The model under review builds one solid part; all positions refer to its coordinate system, in mm. A direction names the side the tool comes from. Give positions to 0.01 mm unless a question says otherwise; leave off trailing zeros. Order: outer loops, then holes, each group sorted by start corner. A loop starts at its lowest first (then second) coordinate and runs counter-clockwise, first axis right, second up. Notation, with made-up numbers: (3.25, 66.25) -> (14.25, 66.25) arc R28 ccw to (14.25, 93.25) -> close; hole circle Ø4 at (66, -18). An arc over 180 degrees is marked (long way). Answer as a JSON object with one key per item and string values. Group by question number.
from build123d import *

# Parameters (mm, degrees)
SKETCH_3_R           = 9.5
CUT_EXTRUDE_1_DEPTH  = 321.526909947
SKETCH_4_R           = 9.5
CUT_EXTRUDE_2_DEPTH  = 321.526909947
SKETCH_5_R           = 9.5
CUT_EXTRUDE_3_DEPTH  = 321.526909947
SKETCH_6_R           = 9.5
CUT_EXTRUDE_4_DEPTH  = 321.526909947
SKETCH_7_R           = 9.5
CUT_EXTRUDE_5_DEPTH  = 321.526909947
SKETCH_8_R           = 9.5
CUT_EXTRUDE_6_DEPTH  = 321.526909947
SKETCH_9_R           = 9.5
CUT_EXTRUDE_7_DEPTH  = 321.526909947
SKETCH_10_R          = 9.5
CUT_EXTRUDE_8_DEPTH  = 321.526909947
SKETCH_11_R          = 9.5
CUT_EXTRUDE_9_DEPTH  = 321.526909947
SKETCH_12_R          = 9.5
CUT_EXTRUDE_10_DEPTH = 321.526909947
SKETCH_13_R          = 9.5
CUT_EXTRUDE_11_DEPTH = 321.526909947
SKETCH_14_R          = 9.5
CUT_EXTRUDE_12_DEPTH = 321.526909947


with BuildPart() as part:
    # Эскиз1 → Повернуть1 (revolve)
    with BuildSketch(Plane.XY, mode=Mode.PRIVATE) as revolve_1_sk:
        Polygon((0, 0), (265, 0), (265, 127.5), (239, 127.5), (239, 100), (239, 95), (220, 95), (220, 94), (200, 94), (144, 65.5), (70, 65.5), (25, 41), (1.5, 41), (3, 45), (0, 45), align=None)
    revolve(revolve_1_sk.sketch.rotate(Axis((0, 0, 0), (1, 0, 0)), 90), axis=Axis((0, 0, 0), (1, 0, 0)))

    # Эскиз2 → Вырез-Повернуть1 (revolve, cut)
    with BuildSketch(Plane.XY, mode=Mode.PRIVATE) as cut_revolve_1_sk:
        with BuildLine():
            Line((0, 0), (200, 0))
            Line((200, 0), (200, 55))
            Line((200, 55), (192.669873, 55))
            ThreePointArc((192.669873, 55), (191.273625348, 54.108499061), (191.669873, 52.5))
            Line((191.669873, 52.5), (188.5, 52.5))
            ThreePointArc((188.5, 52.5), (187.75, 52.602347572), (187, 52.5))
            Line((187, 52.5), (177, 52.5))
            Line((177, 52.5), (95, 52.5))
            Line((95, 52.5), (90, 52.5))
            ThreePointArc((90, 52.5), (79.13262933, 46.740617582), (70, 38.502577))
            Line((70, 38.502577), (42, 31))
            Line((42, 31), (0, 31))
            Line((0, 31), (0, 0))
        make_face()
    revolve(cut_revolve_1_sk.sketch.rotate(Axis((0, 0, 0), (1, 0, 0)), 90), axis=Axis((0, 0, 0), (1, 0, 0)), mode=Mode.SUBTRACT)

    # Эскиз3 → Вырез-Вытянуть1 (cut, through all)
    with BuildSketch(Plane(origin=(0, 0, 0), x_dir=(0, 0, -1), z_dir=(1, 0, 0))):
        with Locations((0, 113)):
            Circle(SKETCH_3_R)
    extrude(amount=CUT_EXTRUDE_1_DEPTH, mode=Mode.SUBTRACT)

    # Эскиз4 → Вырез-Вытянуть2 (cut, through all)
    with BuildSketch(Plane(origin=(0, 0, 0), x_dir=(0, 0, -1), z_dir=(1, 0, 0))):
        with Locations((-56.5, 97.860870628)):
            Circle(SKETCH_4_R)
    extrude(amount=CUT_EXTRUDE_2_DEPTH, mode=Mode.SUBTRACT)

    # Эскиз5 → Вырез-Вытянуть3 (cut, through all)
    with BuildSketch(Plane(origin=(0, 0, 0), x_dir=(0, 0, -1), z_dir=(1, 0, 0))):
        with Locations((-97.860870628, 56.5)):
            Circle(SKETCH_5_R)
    extrude(amount=CUT_EXTRUDE_3_DEPTH, mode=Mode.SUBTRACT)

    # Эскиз6 → Вырез-Вытянуть4 (cut, through all)
    with BuildSketch(Plane(origin=(0, 0, 0), x_dir=(0, 0, -1), z_dir=(1, 0, 0))):
        with Locations((-113, 0)):
            Circle(SKETCH_6_R)
    extrude(amount=CUT_EXTRUDE_4_DEPTH, mode=Mode.SUBTRACT)

    # Эскиз7 → Вырез-Вытянуть5 (cut, through all)
    with BuildSketch(Plane(origin=(0, 0, 0), x_dir=(0, 0, -1), z_dir=(1, 0, 0))):
        with Locations((-97.860870628, -56.5)):
            Circle(SKETCH_7_R)
    extrude(amount=CUT_EXTRUDE_5_DEPTH, mode=Mode.SUBTRACT)

    # Эскиз8 → Вырез-Вытянуть6 (cut, through all)
    with BuildSketch(Plane(origin=(0, 0, 0), x_dir=(0, 0, -1), z_dir=(1, 0, 0))):
        with Locations((-56.5, -97.860870628)):
            Circle(SKETCH_8_R)
    extrude(amount=CUT_EXTRUDE_6_DEPTH, mode=Mode.SUBTRACT)

    # Эскиз9 → Вырез-Вытянуть7 (cut, through all)
    with BuildSketch(Plane(origin=(0, 0, 0), x_dir=(0, 0, -1), z_dir=(1, 0, 0))):
        with Locations((0, -113)):
            Circle(SKETCH_9_R)
    extrude(amount=CUT_EXTRUDE_7_DEPTH, mode=Mode.SUBTRACT)

    # Эскиз10 → Вырез-Вытянуть8 (cut, through all)
    with BuildSketch(Plane(origin=(0, 0, 0), x_dir=(0, 0, -1), z_dir=(1, 0, 0))):
        with Locations((56.5, -97.860870628)):
            Circle(SKETCH_10_R)
    extrude(amount=CUT_EXTRUDE_8_DEPTH, mode=Mode.SUBTRACT)

    # Эскиз11 → Вырез-Вытянуть9 (cut, through all)
    with BuildSketch(Plane(origin=(0, 0, 0), x_dir=(0, 0, -1), z_dir=(1, 0, 0))):
        with Locations((97.860870628, -56.5)):
            Circle(SKETCH_11_R)
    extrude(amount=CUT_EXTRUDE_9_DEPTH, mode=Mode.SUBTRACT)

    # Эскиз12 → Вырез-Вытянуть10 (cut, through all)
    with BuildSketch(Plane(origin=(0, 0, 0), x_dir=(0, 0, -1), z_dir=(1, 0, 0))):
        with Locations((113, 0)):
            Circle(SKETCH_12_R)
    extrude(amount=CUT_EXTRUDE_10_DEPTH, mode=Mode.SUBTRACT)

    # Эскиз13 → Вырез-Вытянуть11 (cut, through all)
    with BuildSketch(Plane(origin=(0, 0, 0), x_dir=(0, 0, -1), z_dir=(1, 0, 0))):
        with Locations((97.860870628, 56.5)):
            Circle(SKETCH_13_R)
    extrude(amount=CUT_EXTRUDE_11_DEPTH, mode=Mode.SUBTRACT)

    # Эскиз14 → Вырез-Вытянуть12 (cut, through all)
    with BuildSketch(Plane(origin=(0, 0, 0), x_dir=(0, 0, -1), z_dir=(1, 0, 0))):
        with Locations((56.5, 97.860870628)):
            Circle(SKETCH_14_R)
    extrude(amount=CUT_EXTRUDE_12_DEPTH, mode=Mode.SUBTRACT)


solid = part.part
1. Draft analysis for pull direction X (two halves, no side actions). For faces 1 (the cylindrical face through (251.82, 56.92, 107.35)), 2 (the conical face through (1.594, 25.1, -32.735)), 3 (the flat face through (265, -2, 2)), state which applies: pulls with the +X half, pulls with the -X half, needs draft (parallel to the pull), parting line crosses it, or undercut.
2. Machinability: for faces 4 (the cylindrical face through (251.82, 124.47, -27.64)), 5 (the conical face through (27.185, 41.186, -9.146)), 6 (the cylindrical face through (20.706, -30.736, -4.036)), which of the approach directions +Z, -Z, +X, -X, +Y, -Y give a long, thin tool a straight path to every point of the face, cutting with its end or side? Answer none if there is none.
3. Take a section at A-A on y = -113. Give the boundary of the cut face in (x, z).
4. Take a section at C-C on y = 0. State how many separate pieces and enclosed holes the cut face has, plus the area to 3 significant figures.
5. Take a section at B-B on x = 17. Give the boundary of the cut face in (y, z).
6. Take a section at D-D on x = 206.5. Give the boundary of the cut face in (y, z), plus the area to 3 significant figures.
7. For pin 1 (17 mm diameter, centred on y = -97.86, z = -56.5, fed in from +X); pin 2 (1.5 mm diameter, centred on x = 32.5, z = 21.5, fed in from -Y); pin 3 (3 mm diameter, centred on y = -86, z = -52.5, fed in from -X); pin 4 (8 mm diameter, centred on x = 30.5, y = 20, fed in from +Z), all flat-tipped, find the tip position at first contact; note any pin that passes through.
8. For probe 1 along X at (y, z) = (33, -30); probe 2 along Y at (x, z) = (115, 0); probe 3 along X at (y, z) = (-71.5, -82), list the stretches that pass through material, from the lowest coordinate up. Write a range as [from, to].
Checks:
{
 "1": {"face 1": "needs draft", "face 2": "undercut", "face 3": "pulls with the +X half"},
 "2": {"face 4": "+X, -X", "face 5": "none", "face 6": "-X"},
 "3": {"outline": "(239, -59.05) -> (265, -59.05) -> (265, -9.5) -> (239, -9.5) -> close; (239, 9.5) -> (265, 9.5) -> (265, 59.05) -> (239, 59.05) -> close"},
 "4": {"separate pieces": "3", "enclosed holes": "0", "area": "20,500 mm2"},
 "5": {"outline": "circle Ø82 at (0, 0); hole circle Ø62 at (0, 0)"},
 "6": {"outline": "circle Ø188 at (0, 0)", "area": "27,800 mm2"},
 "7": {"pin 1": "passes through", "pin 2": "stops at y = -40.24", "pin 3": "stops at x = 239", "pin 4": "stops at z = 42.22"},
 "8": {"probe 1": "x = [0, 2.85], [31.61, 76.29], [200, 265]", "probe 2": "y = [-65.5, -52.5], [52.5, 65.5]", "probe 3": "x = [239, 265]"}
}
